The figure shows three views and two pictorial views of one solid part (mm, origin at its lowest corner). Answer the questions. A direction names the side the tool comes from. Coordinates: 2 decimals unless noted, no trailing zeros. Loops run counter-clockwise (first coordinate to the right, second up) from the corner with the lowest first, then second, coordinate; pieces in that order, holes last. Notation, with made-up numbers: (-38.5, -20.75) -> (-24.5, -20.75) arc R23 cw to (-24.5, 16.25) -> close; hole circle Ø3 at (40.25, 78.5). An arc over 180 degrees is marked (long way). Answer as a JSON object with one key per item and string values. Group by question number.
1) Which of the six approach directions +Z, -Z, +X, -X, +Y, -Y give full straight-line access (tool end or side, diameter ignored) to the marked faces 1 and 2?
2) Consider probe 1 along X at (y, z) = (14.5, 14.75); probe 2 along Z at (x, y) = (48, 9); probe 3 along X at (y, z) = (18.25, 23.5). Determine where each line is inside the solid, lowest interval first. Write a range as [from, to].
3) Section A-A, the plane y = 10.5 is taken. Give the vertices of the cut face in (x, z), plus the area to 3 significant figures.
4) Section B-B, the plane z = 17 is taken. Give the vertices of the cut face in (x, y), plus the area to 3 significant figures.
5) Flat-ended cylindrical pins translate along their axes: P1, Ø3, axis at y = 12, z = 16.5, coming from the +X side; P2, Ø9.5, axis at x = 40, y = 8.5, coming from the +Z side. Find the tip coordinate at first contact, or state that the pin passes through.
6) Section C-C, the plane x = 38.5 is taken. Give the vertices of the cut face in (y, z).
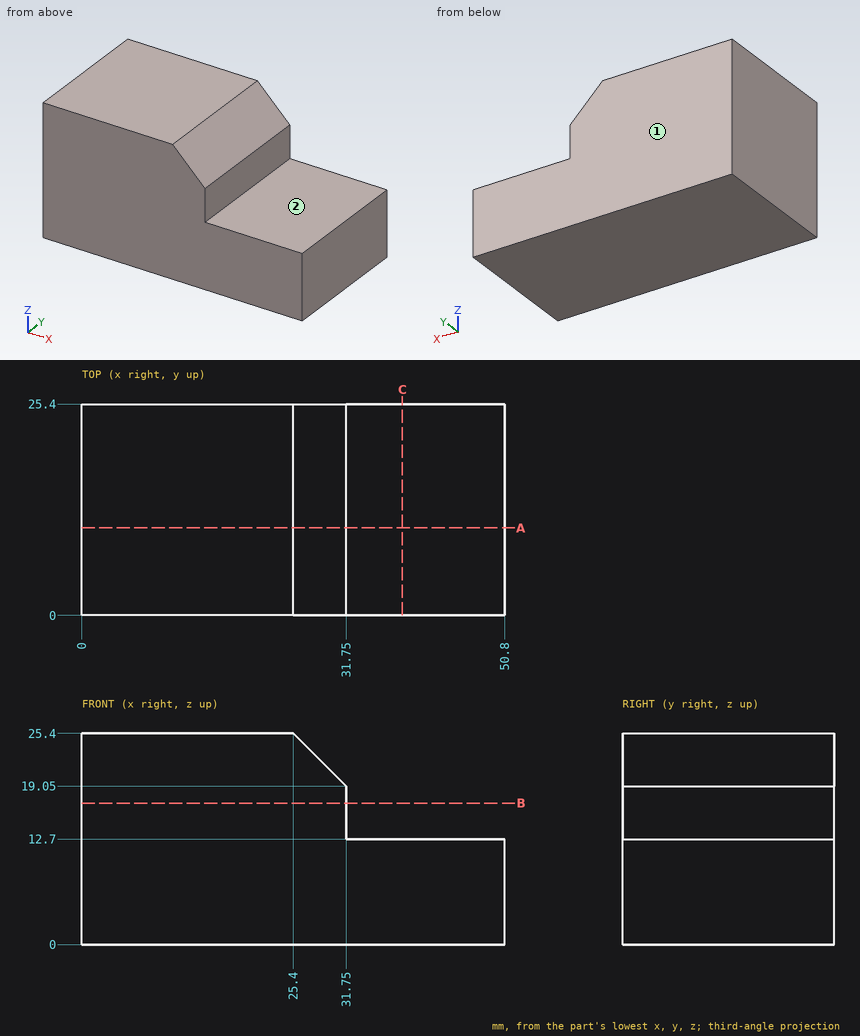
Determined:
{
 "1": {"face 1": "+Z, -Z, +X, -X, +Y", "face 2": "+Z, +X, +Y, -Y"},
 "2": {"probe 1": "[0, 31.75]", "probe 2": "[0, 12.7]", "probe 3": "[0, 27.3]"},
 "3": {"outline": "(0, 0) -> (50.8, 0) -> (50.8, 12.7) -> (31.75, 12.7) -> (31.75, 19.05) -> (25.4, 25.4) -> (0, 25.4) -> close", "area": "1,030 mm²"},
 "4": {"outline": "(0, 0) -> (31.75, 0) -> (31.75, 25.4) -> (0, 25.4) -> close", "area": "806 mm²"},
 "5": {"P1": "x = 31.75", "P2": "z = 12.7"},
 "6": {"outline": "(0, 0) -> (25.4, 0) -> (25.4, 12.7) -> (0, 12.7) -> close"}
}
